Can you work these out from the model? Positions are in its coordinate system, mm. Coordinates: 2 decimals unless noted, no trailing zeros. Loops run counter-clockwise (first coordinate to the right, second up) from the corner with the lowest first, then second, coordinate; pieces in that order, holes last. Notation, with made-up numbers: M 71,29.25 L 85,29.25 A18 cw 85,55.25 Z; hole C 60,31.25 d10. An arc over 180 degrees is marked long. Return JSON: item names as keys, results as strings. Group by question number.
```python
from build123d import *

# Parameters (mm, degrees)
F0_W     = 40
F0_H     = 4
F0_W_2   = 1.9
F0_H_2   = 1.9
F1_DEPTH = 1
F2_W     = 1.9
F2_H     = 1.9
F3_DEPTH = 2
F4_R     = 0.5


with BuildPart() as f1:
    # F0 (on Front) → F1 (new body)
    with BuildSketch(Plane.XZ):
        Rectangle(F0_W, F0_H)
        with Locations((17.95, 0)):
            Rectangle(F0_W_2, F0_H_2, mode=Mode.SUBTRACT)
        with Locations((17.95, 0)):
            Rectangle(F0_W_2, F0_H_2)
    extrude(amount=F1_DEPTH)

    # F2 (on face) → F3 (join)
    with BuildSketch(Plane.XZ.offset(1)):
        with Locations((18, 0)):
            Rectangle(F2_W, F2_H)
    extrude(amount=F3_DEPTH)

    # F4
    f4_edges = [f1.edges().sort_by_distance(p)[0] for p in [
        (18.95, -2, 0.95),
        (17.05, -2, 0.95),
        (18.95, -2, -0.95),
        (17.05, -2, -0.95),
    ]]
    fillet(f4_edges, radius=F4_R)


solid = f1.part
```
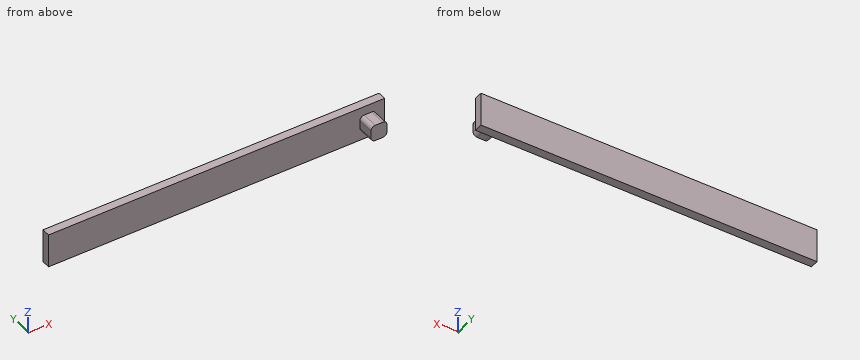
1) If I drill on line 1 (Y direction, x = 9.5, z = 0.7); line 2 (X direction, y = -1.5, z = -0.05); line 3 (X direction, y = -1.7, z = -0.8), over which ranges is the centre line in solid material (lowest first)? Write a range as from..to.
2) Suppose I cut it at A-A, the plane y = -1.95. List the corners of the cut face in (x, z) for me.
3) For pin 1 (1 mm diameter, centred on x = 11, z = 0.5, fed in from -Y); pin 2 (0.5 mm diameter, centred on y = -2, z = 0, fed in from +X); pin 3 (1 mm diameter, centred on y = -2.5, z = 0, fed in from -X), each with a flat end and sliding along its axis, tell me the tip position at first contact or that it passes through.
4) Suppose I cut it at C-C, the plane z = 1.3. List the corners of the cut face in (x, y) for me, then the cut area to 3 significant figures.
5) Suppose I cut it at B-B, the plane x = -16. List the corners of the cut face in (y, z) for me, then the cut area to 3 significant figures.
Returned:
{
 "1": {"line 1": "y = -1..0", "line 2": "x = 17.05..18.95", "line 3": "x = 17.19..18.81"},
 "2": {"outline": "M 17.05,-0.45 A0.5 ccw 17.55,-0.95 L 18.45,-0.95 A0.5 ccw 18.95,-0.45 L 18.95,0.45 A0.5 ccw 18.45,0.95 L 17.55,0.95 A0.5 ccw 17.05,0.45 Z"},
 "3": {"pin 1": "stops at y = -1", "pin 2": "stops at x = 18.95", "pin 3": "stops at x = 17.05"},
 "4": {"outline": "M -20,-1 L 20,-1 L 20,0 L -20,0 Z", "area": "40.0 mm²"},
 "5": {"outline": "M -1,-2 L 0,-2 L 0,2 L -1,2 Z", "area": "4.00 mm²"}
}
